Autodesk Inventor part; units mm, degrees
ref_plane "YZ Plane" through (0, 0, 0) normal (1, 0, 0) x (0, 1, 0)
ref_plane "XZ Plane" through (0, 0, 0) normal (0, 1, 0) x (-1, 0, 0)
ref_plane "XY Plane" through (0, 0, 0) normal (0, 0, 1) x (1, 0, 0)
sketch "Boceto1" plane through (0, 0, 0) normal (0, 1, 0) x (-1, 0, 0)
  line L0 (-41.5, 19.5) -> (41.5, 19.5)
  line L1 (41.5, 19.5) -> (41.5, -19.5)
  line L2 (41.5, -19.5) -> (-41.5, -19.5)
  line L3 (-41.5, -19.5) -> (-41.5, 19.5)
  line L4 (-41.5, 19.5) -> (41.5, -19.5) construction
  line L5 (41.5, 19.5) -> (-41.5, -19.5) construction
  line L6 (-40.5, 18.5) -> (40.5, 18.5)
  line L7 (40.5, 18.5) -> (40.5, -18.5)
  line L8 (40.5, -18.5) -> (-40.5, -18.5)
  line L9 (-40.5, -18.5) -> (-40.5, 18.5)
  line L10 (-40.5, 18.5) -> (40.5, -18.5) construction
  line L11 (40.5, 18.5) -> (-40.5, -18.5) construction
  point P0 (0, 0)
  dimension "d0" = 83
  dimension "d1" = 39
  dimension "d2" = 1
  dimension "d3" = 1
extrude "Extrusión1" add sketch "Boceto1" along normal blind 3 contours L6 L7 L8 L9
extrude "Extrusión2" add sketch "Boceto1" along normal blind 20
sketch "Boceto2" plane through (0, 20, 0) normal (0, 1, 0) x (1, 0, 0)
  line L0 (41.5, 19.5) -> (-41.5, 19.5)
  line L1 (41.5, -19.5) -> (-41.5, -19.5)
  line L2 (-41.5, -19.5) -> (-41.5, 19.5)
  line L3 (-41.5, 19.5) -> (41.5, 19.5)
  line L4 (41.5, 19.5) -> (41.5, -19.5)
  line L5 (41.5, -19.5) -> (-41.5, 19.5) construction
  line L6 (-41.5, -19.5) -> (41.5, 19.5) construction
  line L7 (35.5, -13.5) -> (-35.5, -13.5)
  line L8 (-35.5, -13.5) -> (-35.5, 13.5)
  line L9 (-35.5, 13.5) -> (35.5, 13.5)
  line L10 (35.5, 13.5) -> (35.5, -13.5)
  line L11 (35.5, -13.5) -> (-35.5, 13.5) construction
  line L12 (-35.5, -13.5) -> (35.5, 13.5) construction
  point P0 (0, 0)
  dimension "d8" = 6
  dimension "d9" = 6
extrude "Extrusión3" add sketch "Boceto2" along normal blind 1
sketch "Boceto3" plane through (0, 21, 0) normal (0, 1, 0) x (1, 0, 0)
  point P0 (0, 0)
sketch "Boceto4" plane through (0, 21, 0) normal (0, 1, 0) x (1, 0, 0)
  line L0 (-41.5, 19.5) -> (-41.5, -19.5)
  line L1 (41.5, -19.5) -> (-41.5, -19.5)
  line L2 (-41.5, -19.5) -> (-41.5, 19.5)
  line L3 (-41.5, 19.5) -> (41.5, 19.5)
  line L4 (41.5, 19.5) -> (41.5, -19.5)
  line L5 (41.5, -19.5) -> (-41.5, 19.5) construction
  line L6 (-41.5, -19.5) -> (41.5, 19.5) construction
  line L7 (40.5, -18.5) -> (-40.5, -18.5)
  line L8 (-40.5, -18.5) -> (-40.5, 18.5)
  line L9 (-40.5, 18.5) -> (40.5, 18.5)
  line L10 (40.5, 18.5) -> (40.5, -18.5)
  line L11 (40.5, -18.5) -> (-40.5, 18.5) construction
  line L12 (-40.5, -18.5) -> (40.5, 18.5) construction
  point P0 (0, 0)
  point P1 (-41.5, -19.5)
  dimension "d21" = 1
  dimension "d22" = 1
extrude "Extrusión4" add sketch "Boceto4" along normal blind 32.5
properties part number "Capsula" material "Plástico PET"
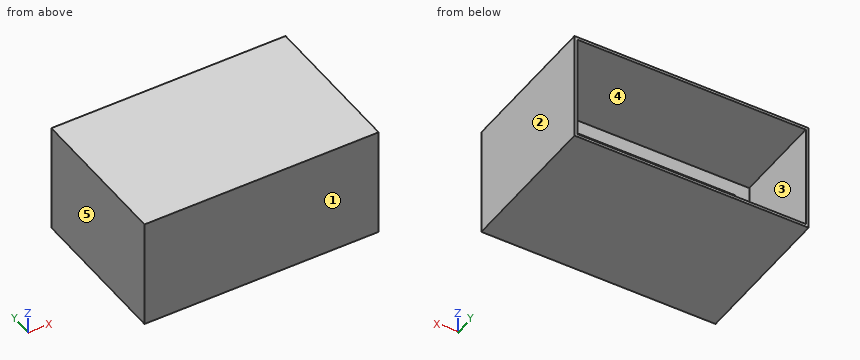
Here's how the part is built. I have some questions about the finished solid (model axes, mm). Face numbers are marked on the shaded views. A direction names the side the tool comes from. Coordinates: 2 decimals unless noted, no trailing zeros. Order: outer loops, then holes, each group sorted by start corner. A loop starts at its lowest first (then second) coordinate and runs counter-clockwise, first axis right, second up. Notation, with made-up numbers: (70.25, 24) - (91.25, 24) arc R22 ccw to (91.25, 32) - close; hole circle Ø7 at (83, 67). An arc over 180 degrees is marked (long way). One line per question, with ' | ' between items.
(1) Suppose I cut it at A-A on y = 43. List the corners of the cut face in (x, z) for me.
Report:
outline: (-41.5, -19.5) - (41.5, -19.5) - (41.5, 19.5) - (-41.5, 19.5) - close; hole (-40.5, -18.5) - (40.5, -18.5) - (40.5, 18.5) - (-40.5, 18.5) - close
(2) If we mould it in two halves opening along X, with no side actions, what happens to the marked faces 1, 2 and 3? For each: pulls with the +X half, pulls with the -X half, needs draft (parallel to the pull), parting line crosses it, or undercut.
Report:
face 1: needs draft | face 2: pulls with the +X half | face 3: undercut
(3) For the marked faces 4 and 5, which set-ups out of +Z, -Z, +X, -X, +Y, -Y let a thin tool reach every point of the face, with its end or its side?
Report:
face 4: +Y | face 5: +Z, -Z, -X, +Y, -Y
(4) Suppose I cut it at C-C on z = -12. List the corners of the cut face in (x, y) for me, and give its area (3 significant figures).
Report:
outline: (-41.5, 0) - (41.5, 0) - (41.5, 53.5) - (40.5, 53.5) - (40.5, 21) - (35.5, 21) - (35.5, 20) - (40.5, 20) - (40.5, 3) - (-40.5, 3) - (-40.5, 20) - (-35.5, 20) - (-35.5, 21) - (-40.5, 21) - (-40.5, 53.5) - (-41.5, 53.5) - close | area: 360 mm2
(5) If I drill on L1, parallel to Z at x = 37, y = 33.5; L2, parallel to X at y = 47, z = 8.5; L3, parallel to Y at x = 0.5, z = 18, over which ranges is the centre line in solid material (lowest first)?
Report:
L1: z = -19.5 to -18.5, 18.5 to 19.5 | L2: x = -41.5 to -40.5, 40.5 to 41.5 | L3: y = 0 to 3, 20 to 21
(6) Will this pin go through, and if not, where does the flat tip stop? pin 1 (18.5 mm diameter, centred on x = 17, z = 3, fed in from +Y).
Report:
pin 1: stops at y = 3
(7) Suppose I cut it at B-B on x = 7. List the corners of the cut face in (y, z) for me, and give its area (3 significant figures).
Report:
outline: (0, -19.5) - (53.5, -19.5) - (53.5, -18.5) - (21, -18.5) - (21, -13.5) - (20, -13.5) - (20, -18.5) - (3, -18.5) - (3, 18.5) - (20, 18.5) - (20, 13.5) - (21, 13.5) - (21, 18.5) - (53.5, 18.5) - (53.5, 19.5) - (0, 19.5) - close | area: 228 mm2
(8) Suppose I cut it at D-D on z = 17. List the corners of the cut face in (x, y) for me, and give its area (3 significant figures).
Report:
outline: (-41.5, 0) - (41.5, 0) - (41.5, 53.5) - (40.5, 53.5) - (40.5, 21) - (-40.5, 21) - (-40.5, 53.5) - (-41.5, 53.5) - close; hole (-40.5, 3) - (40.5, 3) - (40.5, 20) - (-40.5, 20) - close | area: 431 mm2
